```python
from build123d import *

# Parameters (mm, degrees)
F0_R       = 11.176
F1_DEPTH   = 7.62
F2_SIZE2   = 2.1997045256
F2_SIZE    = 3.81
F2_2_SIZE2 = 2.1997045256
F2_2_SIZE  = 3.81
F3_SIZE2   = 2.1997045256
F3_SIZE    = 3.81
F4_SIZE    = 2.54


# Not quite as in the source:
# - a feature names something its author has since deleted; it is built from what else it names


with BuildPart() as f1:
    # F0 (on Top) → F1 (new body)
    with BuildSketch(Plane.XY):
        with BuildLine():
            ThreePointArc((9.7057271537, 23.5283748909), (-0.0208649872, 15.4470615517), (-9.6943160077, 23.5919105566))
            Line((-9.6943160077, 23.5919105566), (-19.3886320155, 27.4654462223))
            Line((-19.3886320155, 27.4654462223), (-24.1059964708, 29.3503527439))
            Line((-24.1059964708, 29.3503527439), (-46.1373193312, 27.748740566))
            Line((-46.1373193312, 27.748740566), (-37.463364806, 6.2451757293))
            Line((-37.463364806, 6.2451757293), (-33.4914395336, 3.0781251091))
            Line((-33.4914395336, 3.0781251091), (-25.3390191684, -3.4222811682))
            ThreePointArc((-25.3390191684, -3.4222811682), (-13.4326493579, -7.7553437227), (-15.6332920147, -20.2330937227))
            Line((-15.6332920147, -20.2330937227), (-14.0799852263, -30.5435))
            Line((-14.0799852263, -30.5435), (-13.3232015704, -35.5668134979))
            Line((-13.3232015704, -35.5668134979), (-0.0898891733, -53.8478470607))
            Line((-0.0898891733, -53.8478470607), (13.3370282377, -35.4750360336))
            Line((13.3370282377, -35.4750360336), (14.0938118937, -30.4517225357))
            Line((14.0938118937, -30.4517225357), (15.6402053484, -20.1872049906))
            ThreePointArc((15.6402053484, -20.1872049906), (13.4326493579, -7.7553437227), (25.3027350274, -3.4512126568))
            Line((25.3027350274, -3.4512126568), (33.4188712518, 3.0202621318))
            Line((33.4188712518, 3.0202621318), (37.3907965242, 6.1873127519))
            Line((37.3907965242, 6.1873127519), (46.633735943, 26.924))
            Line((46.633735943, 26.924), (24.1401632357, 29.1946377686))
            Line((24.1401632357, 29.1946377686), (19.4114543073, 27.3383748909))
            Line((19.4114543073, 27.3383748909), (9.7057271537, 23.5283748909))
        make_face()
        with Locations((0, -27.432)):
            Circle(F0_R, mode=Mode.SUBTRACT)
        Circle(F0_R, mode=Mode.SUBTRACT)
        with Locations((-23.7568088766, 13.716)):
            Circle(F0_R, mode=Mode.SUBTRACT)
        with Locations((23.7568088766, 13.716)):
            Circle(F0_R, mode=Mode.SUBTRACT)
    extrude(amount=F1_DEPTH)

    # F2
    f2_edges = [f1.edges().sort_by_distance(p)[0] for p in [
        (-41.800342, 16.996958, 7.62),
        (-35.121658, 28.549547, 7.62),
        (35.38695, 28.059319, 7.62),
        (42.012266, 16.555656, 7.62),
        (6.62357, -44.661442, 7.62),
        (-6.706545, -44.70733, 7.62),
    ]]
    f2_side = f1.faces().sort_by_distance((13.256392, -27.645481, 7.62))[0]
    chamfer(f2_edges, length=F2_SIZE, length2=F2_SIZE2, reference=f2_side)

    # F2#2
    f2_2_edges = [f1.edges().sort_by_distance(p)[0] for p in [
        (-41.800342, 16.996958, 0),
        (42.012266, 16.555656, 0),
        (-35.121658, 28.549547, 0),
    ]]
    f2_2_side = f1.faces().sort_by_distance((12.353469, -7.132279, 0))[0]
    chamfer(f2_2_edges, length=F2_2_SIZE, length2=F2_2_SIZE2, reference=f2_2_side)

    # F3
    f3_edges = [f1.edges().sort_by_distance(p)[0] for p in [
        (-6.706545, -44.70733, 0),
        (6.62357, -44.661442, 0),
        (33.391083, 28.260794, 0),
    ]]
    f3_side = f1.faces().sort_by_distance((27.377875, -0.292303, 0))[0]
    chamfer(f3_edges, length=F3_SIZE, length2=F3_SIZE2, reference=f3_side)

    # F4
    f4_edges = [f1.edges().sort_by_distance(p)[0] for p in [
        (-0.020865, 15.447062, 7.62),
        (13.432649, -7.755344, 7.62),
        (-13.432649, -7.755344, 7.62),
        (-13.432649, -7.755344, 0),
        (-0.020865, 15.447062, 0),
        (13.432649, -7.755344, 0),
    ]]
    chamfer(f4_edges, length=F4_SIZE)


solid = f1.part
```
Input: part model. Units: mm. Frame: model coordinates. Give positions to 0.01 mm unless a question says otherwise; leave off trailing zeros.
1) Line query: L1, parallel to Y at x = 0, z = 4.75; L2, parallel to X at y = 14.5, z = 2.75; L3, parallel to X at y = 6.5, z = 6.75. Output: solid intervals per line, ascending.
A:
L1: y = -53.72 to -38.61, -16.26 to -11.18, 11.18 to 15.45
L2: x = -40.79 to -34.91, -12.61 to 12.61, 34.91 to 41.1
L3: x = -35.08 to -32.29, -15.22 to -9.09, 9.09 to 15.22, 32.29 to 35.01
2) Mould query, pull axis X, two halves, no side actions, for faces 1 (the flat face through (-38.875, 14.767, 1.115)), 2 (the cylindrical face through (0.17, 15.45, 3.79)), 3 (the flat face through (35.544, 28.043, 3.787)). Classes: released by +X, released by -X, zero draft, split by the parting line, or undercut.
A:
face 1: released by -X
face 2: undercut
face 3: released by +X
3) Section query A-A on y = 19. Count the separate pieces of the cut face and the enclosed holes in it, and give its area (3 significant figures).
A:
separate pieces: 4
enclosed holes: 0
area: 203 mm2
4) Contact query for flat-ended pins moving along their axis: pin 1 (18 mm diameter, centred on x = 0, y = 0, fed in from +Z); pin 2 (1 mm diameter, centred on y = -42, z = 4, fed in from +X); pin 3 (1 mm diameter, centred on x = 11, z = 5.5, fed in from +Y); pin 4 (1 mm diameter, centred on y = -12, z = 2.5, fed in from -X). Output: stop coordinate, or through.
A:
pin 1: passes through
pin 2: stops at x = 8.93
pin 3: stops at y = 24.23
pin 4: stops at x = -12.18
